Input: part model. Units: mm. Frame: model coordinates. A direction names the side the tool comes from. Give positions to 0.01 mm unless a question says otherwise; leave off trailing zeros. Write each loop counter-clockwise with the first axis right and the second up, starting at its lowest first coordinate (ties: lowest second). Pieces come first, ordered by that corner, then holes.
```python
from build123d import *

# Parameters (mm, degrees)
PAD_DEPTH    = 5
CHAMFER_SIZE = 1.5


with BuildPart() as part:
    # Sketch → Pad (new body)
    with BuildSketch(Plane.XY):
        with BuildLine():
            Line((44, 10), (44, 35))
            Line((44, 35), (30, 35))
            Line((30, 35), (30, 10))
            Line((30, 10), (30, 0))
            ThreePointArc((0, 0), (15, -15), (30, 0))
            Line((0, 0), (0, 10))
            ThreePointArc((5, 10), (2.5, 12.5), (0, 10))
            Line((5, 10), (5, 0))
            ThreePointArc((5, 0), (15, -10), (25, 0))
            Line((25, 37.071068), (25, 0))
            Line((27.928932, 40), (25, 37.071068))
            Line((46.071068, 40), (27.928932, 40))
            Line((49, 37.071068), (46.071068, 40))
            Line((49, 10), (49, 37.071068))
            Line((44, 10), (49, 10))
        make_face()
    extrude(amount=PAD_DEPTH)

    # Chamfer
    chamfer_edges = [part.edges().sort_by_distance(p)[0] for p in [
        (44, 22.5, 5),
        (37, 35, 5),
        (30, 17.5, 5),
        (15, -15, 5),
        (0, 5, 5),
        (2.5, 12.5, 5),
        (5, 5, 5),
        (15, -10, 5),
        (25, 18.535534, 5),
        (26.464466, 38.535534, 5),
        (37, 40, 5),
        (47.535534, 38.535534, 5),
        (49, 23.535534, 5),
        (46.5, 10, 5),
        (44, 10, 2.5),
        (49, 10, 2.5),
        (46.5, 10, 0),
        (44, 22.5, 0),
        (37, 35, 0),
        (30, 17.5, 0),
        (15, -15, 0),
        (0, 5, 0),
        (2.5, 12.5, 0),
        (5, 5, 0),
        (15, -10, 0),
        (25, 18.535534, 0),
        (26.464466, 38.535534, 0),
        (37, 40, 0),
        (47.535534, 38.535534, 0),
        (49, 23.535534, 0),
    ]]
    chamfer(chamfer_edges, length=CHAMFER_SIZE)


solid = part.part
```
Item 1: Pin query (flat end, axial travel): pin 1 (1.6 mm diameter, centred on x = 47, z = 2.5, fed in from -Y); pin 2 (1.6 mm diameter, centred on y = 20.5, z = 2, fed in from -X); pin 3 (8 mm diameter, centred on x = 21.5, y = 28, fed in from -Z); pin 4 (1.5 mm diameter, centred on x = 31.5, y = 30, fed in from +Z). Return the tip coordinate at first contact, or that it passes through.
Item 2: Set-up query: faces 4 (the flat face through (25.8, 18.3, 4.3)), 5 (the flat face through (37.1, 35.8, 4.3)), 6 (the flat face through (46, 10, 2)). Return all of +Z, -Z, +X, -X, +Y, -Y with unobstructed straight access to the full face (end or side cutting, diameter ignored); none if empty.
Item 3: Ray query, line 1 (X direction, y = 22, z = 3.3); line 2 (X direction, y = 1, z = 2.8); line 3 (Y direction, x = 46, z = 2.55). Return the intervals inside material, ascending.
Item 4: Section B-B (z = 2.45). Return loops of the section in (x, y).
Item 5: Section C-C (x = 36.5). Return loops of the section in (y, z).
Item 6: Mould query, pull axis X, two halves, no side actions, for faces 1 (the flat face through (48, 11, 1)), 2 (the flat face through (45, 11, 4)), 3 (the flat face through (28, 13, 5)). Classes: +X half, -X half, draft (parallel to the pull), parting line (faces both ways), or undercut.
Item 7: Section A-A (y = 22). Return loops of the section in (x, z).
Solved:
1. pin 1: stops at y = 10
1. pin 2: stops at x = 25
1. pin 3: stops at z = 1
1. pin 4: passes through
2. face 4: +Z, +Y
2. face 5: +Z, -Y
2. face 6: +Z, -Z, +X, -Y
3. line 1: x = 25 to 30, 44 to 49
3. line 2: x = 0 to 5, 25 to 30
3. line 3: y = 10 to 40
4. outline: (0, 0) arc R15 ccw to (30, 0) - (30, 35) - (44, 35) - (44, 11.5) - (45.5, 10) - (47.5, 10) - (49, 11.5) - (49, 37.07) - (46.07, 40) - (27.93, 40) - (25, 37.07) - (25, 0) arc R10 cw to (5, 0) - (5, 10) arc R2.5 ccw to (0, 10) - close
5. outline: (35, 1.5) - (36.5, 0) - (38.5, 0) - (40, 1.5) - (40, 3.5) - (38.5, 5) - (36.5, 5) - (35, 3.5) - close
6. face 1: +X half
6. face 2: undercut
6. face 3: draft
7. outline: (25, 1.5) - (26.5, 0) - (28.5, 0) - (30, 1.5) - (30, 3.5) - (28.5, 5) - (26.5, 5) - (25, 3.5) - close; (44, 1.5) - (45.5, 0) - (47.5, 0) - (49, 1.5) - (49, 3.5) - (47.5, 5) - (45.5, 5) - (44, 3.5) - close
